Verification items for this drawing (mm, ordinates from the low corner). Round coordinates to 2 decimals unless told otherwise and drop trailing zeros. Write each loop counter-clockwise with the first axis right and the second up, starting at its lowest first coordinate (ties: lowest second). Pieces come first, ordered by that corner, then holes. Notation, with made-up numbers: M -17,23.25 L 19,23.25 A24 cw 19,48.25 Z; hole C 74.25,20.25 d3. An arc over 180 degrees is marked long. One line per question, with ' | ' between items. Start each with the question number.
Q1. Cross-section at C-C (z = 11.25). Record the boundary of the cut face in (x, y), then the cut area to 3 significant figures.
Q2. Gauge pin test, flat ends, axial feed: pin 1 (1.5 mm diameter, centred on x = 3.5, z = 6.5, fed in from +Y); pin 2 (2 mm diameter, centred on y = 1, z = 4, fed in from -X). Record the tip position at first contact, or that the pin passes through.
Q3. Cross-section at A-A (x = 2.5). Record the boundary of the cut face in (y, z).
Q4. Thickness scan on line 1 along Y through (x, z) = (2.5, 2.5); line 2 along Y through (x, z) = (1.25, 2). Record the ranges inside material, lowest first. Write a range as from..to.
Q5. Release check for a two-part mould opening along Z. For the marked faces 1, 2 and 3 record: released by +Z, released by -Z, zero draft, split by the parting line, or undercut.
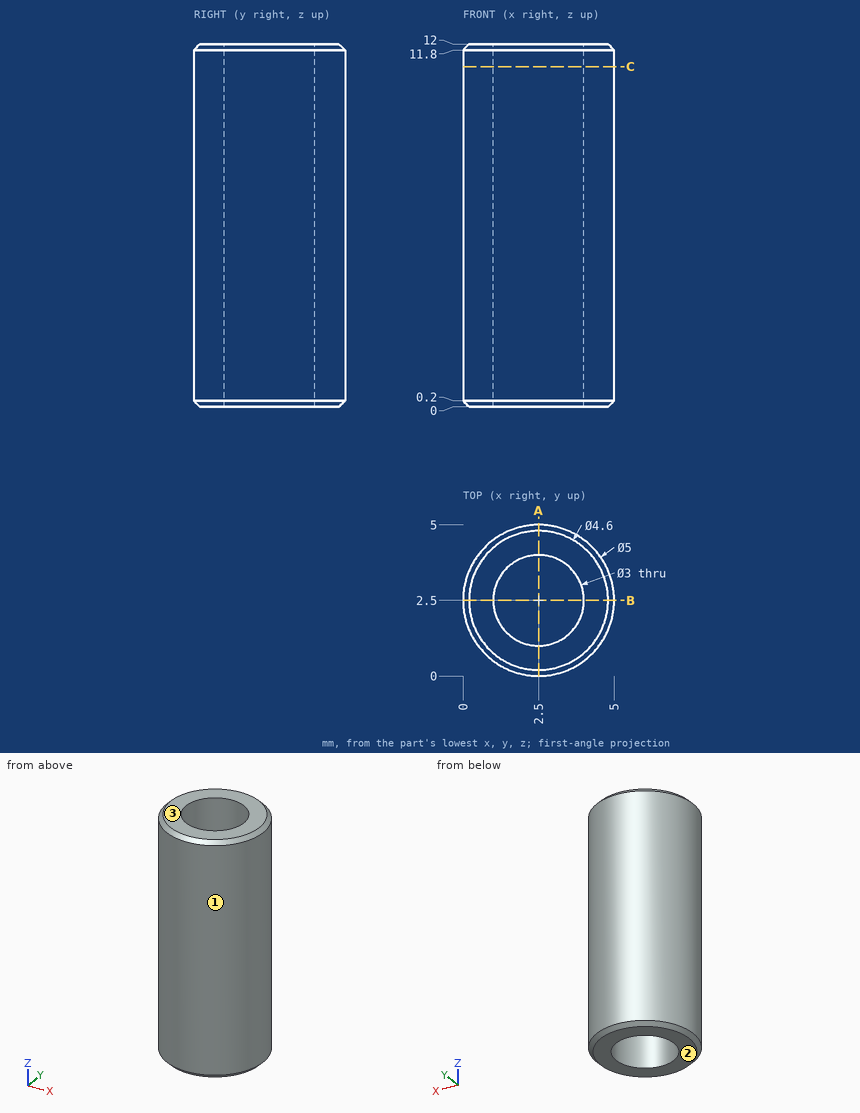
Determined:
1) outline: C 2.5,2.5 d5; hole C 2.5,2.5 d3 | area: 12.6 mm²
2) pin 1: stops at y = 4.99 | pin 2: stops at x = 0.05
3) outline: M 0,0.2 L 0.2,0 L 1,0 L 1,12 L 0.2,12 L 0,11.8 Z; M 4,0 L 4.8,0 L 5,0.2 L 5,11.8 L 4.8,12 L 4,12 Z
4) line 1: y = 0..1, 4..5 | line 2: y = 0.33..1.67, 3.33..4.67
5) face 1: zero draft | face 2: released by -Z | face 3: released by +Z
